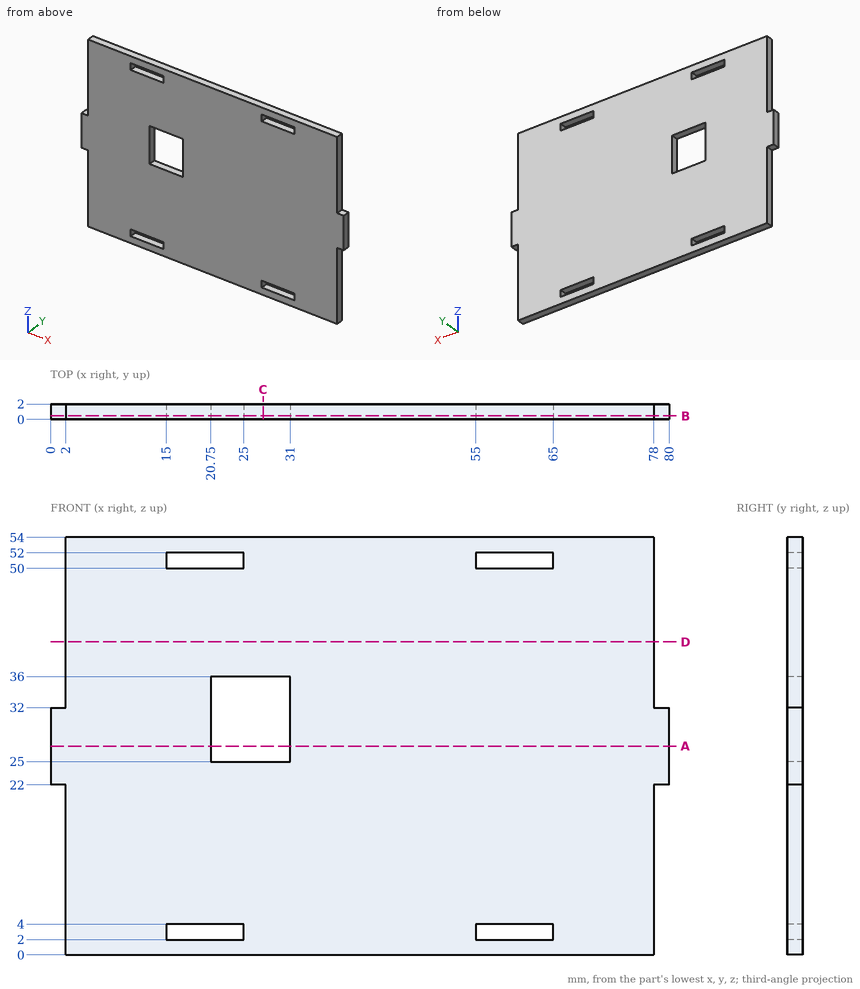
Print and shaded views of the part. All mm, measured from the part's lowest x, y and z. Round coordinates to 2 decimals unless told otherwise and drop trailing zeros. Write each loop counter-clockwise with the first axis right and the second up, starting at its lowest first coordinate (ties: lowest second). Pieces come first, ordered by that corner, then holes. Notation, with made-up numbers: (-7.5, 58) - (1.5, 58) arc R27 ccw to (1.5, 92) - close; hole circle Ø9 at (17.25, 63.25). An arc over 180 degrees is marked (long way). Write each question's results on one line, items separated by ' | '. Start each with the question number.
Item 1: Drop flat-ended pins along their axis: P1, Ø0.6, axis at y = 0.5, z = 51, coming from the -X side; P2, Ø1, axis at y = 0.5, z = 50.5, coming from the +X side. Give the stop position or say it passes through.
Item 2: Saw through at A-A (z = 27). Write the cut outline in (x, y).
Item 3: Saw through at C-C (x = 27.5). Write the cut outline in (y, z), and give its area (3 significant figures).
Item 4: Saw through at B-B (y = 0.45). State how many separate pieces and enclosed holes the cut face has, and give its area (3 significant figures).
Item 5: Saw through at D-D (z = 40.5). Write the cut outline in (x, y), and give its area (3 significant figures).
Item 6: Wall check: L1, parallel to Z at x = 21, y = 1.6; L2, parallel to Z at x = 62, y = 0.8; L3, parallel to X at y = 0.75, z = 51. Give the ranges that are in metal, low to high. Write a range as [from, to].
Results are:
1) P1: stops at x = 2 | P2: stops at x = 78
2) outline: (0, 0) - (20.75, 0) - (20.75, 2) - (0, 2) - close; (31, 0) - (80, 0) - (80, 2) - (31, 2) - close
3) outline: (0, 0) - (2, 0) - (2, 25) - (0, 25) - close; (0, 36) - (2, 36) - (2, 54) - (0, 54) - close | area: 86.0 mm²
4) separate pieces: 1 | enclosed holes: 5 | area: 3,950 mm²
5) outline: (2, 0) - (78, 0) - (78, 2) - (2, 2) - close | area: 152 mm²
6) L1: z = [0, 2], [4, 25], [36, 50], [52, 54] | L2: z = [0, 2], [4, 50], [52, 54] | L3: x = [2, 15], [25, 55], [65, 78]
